For this review, take the finished solid that the model builds, in its own axes (mm). A direction names the side the tool comes from. Round coordinates to 2 decimals unless told otherwise and drop trailing zeros. Order: outer loops, then holes, each group sorted by start corner. A loop starts at its lowest first (then second) coordinate and runs counter-clockwise, first axis right, second up.
```python
from build123d import *

# Parameters (mm, degrees)
SKETCH1_R           = 38.1
BOSS_EXTRUDE1_DEPTH = 12.7
SKETCH3_R           = 44.45
BOSS_EXTRUDE2_DEPTH = 12.7
SKETCH4_R           = 9.144
CUT_EXTRUDE1_DEPTH  = 26.4
SKETCH5_W           = 30.48
SKETCH5_H           = 30.48
CUT_EXTRUDE2_DEPTH  = 17.78
SKETCH6_R           = 31.75
CUT_EXTRUDE3_DEPTH  = 12.7
BOSS_EXTRUDE3_DEPTH = 38.1
CUT_EXTRUDE4_START  = -2.54
SKETCH8_R           = 38.1
SKETCH8_R_2         = 35.052
CUT_EXTRUDE4_DEPTH  = 3.2512
CUT_EXTRUDE5_START  = -7.62
SKETCH9_R           = 38.1
SKETCH9_R_2         = 35.052
CUT_EXTRUDE5_DEPTH  = 3.2512
FILLET1_R           = 2.54
SKETCH10_W          = 35.56
SKETCH10_H          = 35.56
SKETCH10_W_2        = 30.48
SKETCH10_H_2        = 30.48
BOSS_EXTRUDE4_DEPTH = 12.7


with BuildPart() as part:
    # Sketch1 → Boss-Extrude1 (new body)
    with BuildSketch(Plane.XY):
        Circle(SKETCH1_R)
    extrude(amount=BOSS_EXTRUDE1_DEPTH)

    # Sketch3 → Boss-Extrude2 (add)
    with BuildSketch(Plane(origin=(0, 0, 0), x_dir=(-1, 0, 0), z_dir=(0, 0, -1))):
        Circle(SKETCH3_R)
    extrude(amount=BOSS_EXTRUDE2_DEPTH)

    # Sketch4 → Cut-Extrude1 (cut, through all)
    with BuildSketch(Plane(origin=(0, 0, -12.7), x_dir=(-1, 0, 0), z_dir=(0, 0, -1))):
        Circle(SKETCH4_R)
    extrude(amount=-CUT_EXTRUDE1_DEPTH, mode=Mode.SUBTRACT)

    # Sketch5 → Cut-Extrude2 (cut)
    with BuildSketch(Plane.XY.offset(12.7)):
        Rectangle(SKETCH5_W, SKETCH5_H)
    extrude(amount=-CUT_EXTRUDE2_DEPTH, mode=Mode.SUBTRACT)

    # Sketch6 → Cut-Extrude3 (cut)
    with BuildSketch(Plane.XY.offset(12.7)):
        Circle(SKETCH6_R)
    extrude(amount=-CUT_EXTRUDE3_DEPTH, mode=Mode.SUBTRACT)

    # Sketch7 → Boss-Extrude3 (add)
    with BuildSketch(Plane(origin=(0, 0, -12.7), x_dir=(-1, 0, 0), z_dir=(0, 0, -1))):
        with BuildLine():
            Line((-34.21134801, -13.639375622), (-31.460634651, -13.639375622))
            ThreePointArc((-31.460634651, -13.639375622), (0, 34.29), (31.460634651, -13.639375622))
            Line((31.460634651, -13.639375622), (34.21134801, -13.639375622))
            ThreePointArc((34.21134801, -13.639375622), (0, 36.83), (-34.21134801, -13.639375622))
        make_face()
    extrude(amount=BOSS_EXTRUDE3_DEPTH)

    # Sketch8 → Cut-Extrude4 (cut)
    with BuildSketch(Plane.XY.offset(12.7).offset(CUT_EXTRUDE4_START)):
        Circle(SKETCH8_R)
        Circle(SKETCH8_R_2, mode=Mode.SUBTRACT)
    extrude(amount=-CUT_EXTRUDE4_DEPTH, mode=Mode.SUBTRACT)

    # Sketch9 → Cut-Extrude5 (cut)
    with BuildSketch(Plane.XY.offset(12.7).offset(CUT_EXTRUDE5_START)):
        Circle(SKETCH9_R)
        Circle(SKETCH9_R_2, mode=Mode.SUBTRACT)
    extrude(amount=-CUT_EXTRUDE5_DEPTH, mode=Mode.SUBTRACT)

    # Fillet1
    fillet1_edges = [part.edges().sort_by_distance(p)[0] for p in [
        (0, 36.83, -12.7),
        (32.835991331, -13.639375622, -12.7),
        (0, 34.29, -12.7),
        (-32.835991331, -13.639375622, -12.7),
    ]]
    fillet(fillet1_edges, radius=FILLET1_R)

    # Sketch10 → Boss-Extrude4 (add)
    with BuildSketch(Plane.XY):
        Rectangle(SKETCH10_W, SKETCH10_H)
        Rectangle(SKETCH10_W_2, SKETCH10_H_2, mode=Mode.SUBTRACT)
    extrude(amount=BOSS_EXTRUDE4_DEPTH)


solid = part.part
```
Q1. Mouldability with a two-part tool opening along X and no side actions: class faces 5 (the face through (-15.24, 0, 4)), 6 (the face through (17, -31, 1.829)), 7 (the face through (-42.397, 13.352, -6.261)) as +X half, -X half, draft (parallel to the pull), parting line (faces both ways), or undercut.
Q2. Wall thickness on line 1 (Z direction, x = -6.5, y = 34.5); line 2 (Y direction, x = 0, z = 7); line 3 (Z direction, x = 29.5, y = -22): over which ranges is each line inside the solid? List them lowest first.
Q3. Take a section at A-A, the plane z = -1.5. State the section outline as (x, y) points, plus the area to 3 significant figures.
Q4. Take a section at B-B, the plane z = -44. State the section outline as (x, y) points, plus the area to 3 significant figures.
Q5. Clearance check with flat-ended pins moving along their axes: pin 1 (12 mm diameter, centred on x = 3.5, z = 3, fed in from -Y); pin 2 (3 mm diameter, centred on y = 17.5, z = -1.5, fed in from +X); pin 3 (4 mm diameter, centred on y = -11.5, z = -14, fed in from +X). State where each tip first meets the part, or that it passes through.
Q6. Tool access review of faces 1 (the face through (0.95, 34.277, -32.771)), 2 (the face through (-33, -13.639, -33)), 3 (the face through (1.982, -8.927, -8.943)), 4 (the face through (-30.235, -23.183, 0.902)): name each direction out of +Z, -Z, +X, -X, +Y, -Y from which nothing blocks a thin tool from reaching the whole face with its end or side.
Working result:
1. face 5: undercut
1. face 6: draft
1. face 7: parting line
2. line 1: z = -50.8 to 1.83, 5.08 to 6.91, 10.16 to 12.7
2. line 2: y = -35.05 to -31.75, -17.78 to -15.24, 15.24 to 17.78, 31.75 to 35.05
2. line 3: z = -12.7 to 1.83, 5.08 to 6.91, 10.16 to 12.7
3. outline: circle Ø88.9 at (0, 0); hole (-15.24, -15.24) - (15.24, -15.24) - (15.24, 15.24) - (-15.24, 15.24) - close
3. area: 5,280 mm2
4. outline: (-34.21, -13.64) - (-31.46, -13.64) arc R34.29 cw (long way) to (31.46, -13.64) - (34.21, -13.64) arc R36.83 ccw (long way) to start
4. area: 355 mm2
5. pin 1: stops at y = -44.45
5. pin 2: stops at x = 41.47
5. pin 3: stops at x = 43.32
6. face 1: -Z
6. face 2: -Z, +X, -X, -Y
6. face 3: +Z, -Z
6. face 4: +Z
